```python
from build123d import *

# Parameters (mm, degrees)
SKETCH1_W               = 233.68
SKETCH1_H               = 185.42
BOSS_EXTRUDE1_DEPTH     = 2.286
CUT_EXTRUDE1_DEPTH      = 150.170893595
F_1_4_CLEARANCE_HOLE2_D = 6.7564
FILLET1_R               = 12.7
SKETCH9_R               = 2.5527
CUT_EXTRUDE2_DEPTH      = 150.170893595
CUT_EXTRUDE3_DEPTH      = 150.170893595
FILLET2_R               = 1.5875


with BuildPart() as part:
    # Sketch1 → Boss-Extrude1 (new body)
    with BuildSketch(Plane.XY):
        Rectangle(SKETCH1_W, SKETCH1_H)
        with BuildLine():
            Line((-86.36, 16.51), (86.36, 16.51))
            ThreePointArc((86.36, 16.51), (89.952102448, 15.022102448), (91.44, 11.43))
            Line((91.44, 11.43), (91.44, -62.23))
            ThreePointArc((91.44, -62.23), (89.952102448, -65.822102448), (86.36, -67.31))
            Line((86.36, -67.31), (-86.36, -67.31))
            ThreePointArc((-86.36, -67.31), (-89.952102448, -65.822102448), (-91.44, -62.23))
            Line((-91.44, -62.23), (-91.44, 11.43))
            ThreePointArc((-91.44, 11.43), (-89.952102448, 15.022102448), (-86.36, 16.51))
        make_face(mode=Mode.SUBTRACT)
    extrude(amount=BOSS_EXTRUDE1_DEPTH)

    # Sketch2 → Cut-Extrude1 (cut, through all)
    with BuildSketch(Plane.XY.offset(2.286)):
        with BuildLine():
            Line((38.1, 22.225), (-38.1, 22.225))
            ThreePointArc((-38.1, 22.225), (-41.275, 25.4), (-38.1, 28.575))
            Line((-38.1, 28.575), (38.1, 28.575))
            ThreePointArc((38.1, 28.575), (41.275, 25.4), (38.1, 22.225))
        make_face()
        with BuildLine():
            Line((38.1, -73.025), (-38.1, -73.025))
            ThreePointArc((-38.1, -73.025), (-41.275, -76.2), (-38.1, -79.375))
            Line((-38.1, -79.375), (38.1, -79.375))
            ThreePointArc((38.1, -79.375), (41.275, -76.2), (38.1, -73.025))
        make_face()
    extrude(amount=-CUT_EXTRUDE1_DEPTH, mode=Mode.SUBTRACT)

    # 1/4 Clearance Hole2 (through all)
    with Locations(Plane.XY.offset(2.286)):
        with Locations((-38.1, 80.01), (38.1, 80.01)):
            Hole(F_1_4_CLEARANCE_HOLE2_D / 2)

    # Fillet1
    fillet1_edges = [part.edges().sort_by_distance(p)[0] for p in [
        (116.84, -92.71, 1.143),
        (-116.84, -92.71, 1.143),
        (-116.84, 92.71, 1.143),
        (116.84, 92.71, 1.143),
    ]]
    fillet(fillet1_edges, radius=FILLET1_R)

    # Sketch9 → Cut-Extrude2 (cut, through all)
    with BuildSketch(Plane.XY.offset(2.286)):
        with Locations((-104.14, -60.96)):
            Circle(SKETCH9_R)
        with Locations((104.14, -60.96)):
            Circle(SKETCH9_R)
        with Locations((104.14, -35.56)):
            Circle(SKETCH9_R)
        with Locations((-104.14, -35.56)):
            Circle(SKETCH9_R)
    extrude(amount=-CUT_EXTRUDE2_DEPTH, mode=Mode.SUBTRACT)

    # Sketch10 → Cut-Extrude3 (cut, through all)
    with BuildSketch(Plane.XY.offset(2.286)):
        Polygon((-59.06381265, 67.31), (-85.71618735, 67.31), (-72.39, 58.4258751), align=None)
        Polygon((-78.11381265, 54.61), (-91.44, 63.4941249), (-91.44, 45.7258751), align=None)
        Polygon((-59.06381265, 41.91), (-72.39, 50.7941249), (-85.71618735, 41.91), align=None)
        Polygon((-53.34, 63.4941249), (-66.66618735, 54.61), (-53.34, 45.7258751), align=None)
        Polygon((85.71618735, 41.91), (72.39, 50.7941249), (59.06381265, 41.91), align=None)
        Polygon((66.66618735, 54.61), (53.34, 63.4941249), (53.34, 45.7258751), align=None)
        Polygon((85.71618735, 67.31), (59.06381265, 67.31), (72.39, 58.4258751), align=None)
        Polygon((91.44, 63.4941249), (78.11381265, 54.61), (91.44, 45.7258751), align=None)
    extrude(amount=-CUT_EXTRUDE3_DEPTH, mode=Mode.SUBTRACT)

    # Fillet2
    fillet2_edges = [part.edges().sort_by_distance(p)[0] for p in [
        (-72.39, 58.4258751, 1.143),
        (-85.71618735, 67.31, 1.143),
        (-59.06381265, 67.31, 1.143),
        (-91.44, 45.7258751, 1.143),
        (-91.44, 63.4941249, 1.143),
        (-78.11381265, 54.61, 1.143),
        (-85.71618735, 41.91, 1.143),
        (-72.39, 50.7941249, 1.143),
        (-59.06381265, 41.91, 1.143),
        (-66.66618735, 54.61, 1.143),
        (-53.34, 63.4941249, 1.143),
        (-53.34, 45.7258751, 1.143),
        (72.39, 50.7941249, 1.143),
        (85.71618735, 41.91, 1.143),
        (59.06381265, 41.91, 1.143),
        (53.34, 45.7258751, 1.143),
        (53.34, 63.4941249, 1.143),
        (66.66618735, 54.61, 1.143),
        (59.06381265, 67.31, 1.143),
        (85.71618735, 67.31, 1.143),
        (72.39, 58.4258751, 1.143),
        (78.11381265, 54.61, 1.143),
        (91.44, 63.4941249, 1.143),
        (91.44, 45.7258751, 1.143),
    ]]
    fillet(fillet2_edges, radius=FILLET2_R)


solid = part.part
```
Geometry: final body of the model. Coordinates: model frame, mm. A direction names the side the tool comes from. Coordinates: 2 decimals unless noted, no trailing zeros. Order: outer loops, then holes, each group sorted by start corner. A loop starts at its lowest first (then second) coordinate and runs counter-clockwise, first axis right, second up. Notation, with made-up numbers: (30, 84) - (73, 84) arc R15 ccw to (73, 97) - close; hole circle Ø1 at (75.5, 47). An arc over 180 degrees is marked (long way). Return JSON: item names as keys, results as strings. Group by question number.
1. Material intervals for line 1 along Y through (x, z) = (-38.1, 1.35) (3 decimals); line 2 along Y through (x, z) = (-14.5, 1.35) (3 decimals); line 3 along Y through (x, z) = (-104.14, 1.35), sorted ascending. Write a range as [from, to].
2. Pull-direction query (Y, two-part tool) for faces 3 (the face through (-2, 22, 0)), 4 (the face through (38.83, 76.71, 1.13)), 5 (the face through (60.309, 58.848, 1.159)), 6 (the face through (113.02, 89.09, 1.16)); classes: pulls with the +Y half, pulls with the -Y half, needs draft (parallel to the pull), parting line crosses it, or undercut.
3. Set-up query: faces 1 (the face through (113.02, -89.09, 1.16)), 2 (the face through (60.2, 50.3, 1.2)). Return all of +Z, -Z, +X, -X, +Y, -Y with unobstructed straight access to the full face (end or side cutting, diameter ignored); none if empty.
4. Cut plane C-C (y = -76.2). Output: boundary loops of the cut face in (x, z) (3 decimals).
5. Cut plane B-B (x = -11.5). Output: boundary loops of the cut face in (y, z) (3 decimals).
6. Cut plane D-D (z = 1.9). Count the separate pieces of the cut face and the enclosed holes in it, plus the area to 3 significant figures.
7. Cut plane A-A (y = 0.5). Output: boundary loops of the cut face in (x, z), plus the area to 3 significant figures.
Resolved:
{
 "1": {"line 1": "y = [-92.71, -79.375], [-73.025, -67.31], [16.51, 22.225], [28.575, 76.632], [83.388, 92.71]", "line 2": "y = [-92.71, -79.375], [-73.025, -67.31], [16.51, 22.225], [28.575, 92.71]", "line 3": "y = [-92.71, -63.51], [-58.41, -38.11], [-33.01, 92.71]"},
 "2": {"face 3": "needs draft", "face 4": "undercut", "face 5": "undercut", "face 6": "pulls with the +Y half"},
 "3": {"face 1": "+Z, -Z, +X, -Y", "face 2": "+Z, -Z"},
 "4": {"outline": "(-116.84, 0) - (-41.275, 0) - (-41.275, 2.286) - (-116.84, 2.286) - close; (41.275, 0) - (116.84, 0) - (116.84, 2.286) - (41.275, 2.286) - close"},
 "5": {"outline": "(-92.71, 0) - (-79.375, 0) - (-79.375, 2.286) - (-92.71, 2.286) - close; (-73.025, 0) - (-67.31, 0) - (-67.31, 2.286) - (-73.025, 2.286) - close; (16.51, 0) - (22.225, 0) - (22.225, 2.286) - (16.51, 2.286) - close; (28.575, 0) - (92.71, 0) - (92.71, 2.286) - (28.575, 2.286) - close"},
 "6": {"separate pieces": "1", "enclosed holes": "17", "area": "25,800 mm²"},
 "7": {"outline": "(-116.84, 0) - (-91.44, 0) - (-91.44, 2.29) - (-116.84, 2.29) - close; (91.44, 0) - (116.84, 0) - (116.84, 2.29) - (91.44, 2.29) - close", "area": "116 mm²"}
}
